Source: CAD feature listing. Evaluate the final solid. Frame: model axes, mm. Face numbers are marked on the shaded views. Round coordinates to 2 decimals unless told otherwise and drop trailing zeros. Order: outer loops, then holes, each group sorted by start corner. A loop starts at its lowest first (then second) coordinate and runs counter-clockwise, first axis right, second up. Notation, with made-up numbers: M 61.5,-10 L 91.5,-10 A32 cw 91.5,29 Z; hole C 87.25,51 d5. An arc over 180 degrees is marked long. Answer in a Markdown table with one row per item. Add a question column.
```python
from build123d import *

# Parameters (mm, degrees)
F1_DEPTH = 25.4
F2_T     = -2.54
F4_D     = 12.7


with BuildPart() as f1:
    # F0 (on Top) → F1 (new body)
    with BuildSketch(Plane.XY):
        with BuildLine():
            ThreePointArc((-34.137599, 0), (2.286002, -13.83152), (38.709603, 0))
            ThreePointArc((38.709603, 0), (2.286002, 13.957497), (-34.137599, 0))
        make_face()
    extrude(amount=F1_DEPTH)

    # F2
    f2_openings = [f1.faces().sort_by_distance(p)[0] for p in [
        (2.286002, 0.052928, 0),
    ]]
    offset(amount=F2_T, openings=f2_openings)

    # F4 (through all)
    with Locations(Plane(origin=(0, 0, 0), x_dir=(1, 0, 0), z_dir=(0, 0, -1))):
        with Locations((0, 0)):
            Hole(F4_D / 2)


solid = f1.part
```
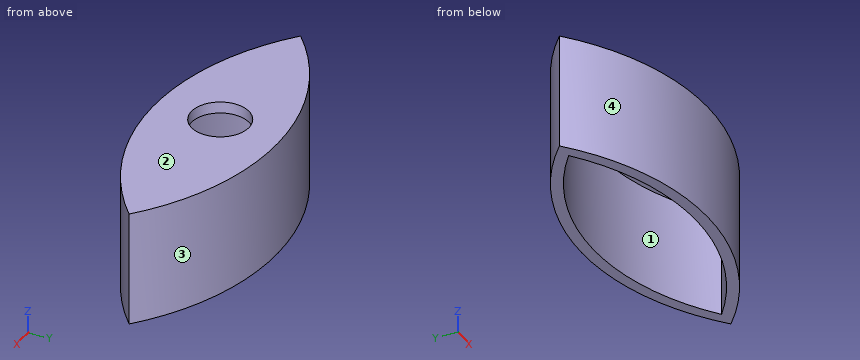
(1) Cut plane A-A (y = 3). Return loops of the section in (x, z), and give its area (3 significant figures).
(2) Cut plane D-D (x = 26). Return loops of the section in (y, z), and give its area (3 significant figures).
(3) Pin query (flat end, axial travel): pin 1 (10 mm diameter, centred on x = -7.5, y = -4.5, fed in from -Z); pin 2 (4 mm diameter, centred on x = 12, z = 13, fed in from -Y); pin 3 (7.5 mm diameter, centred on x = 0, y = 0, fed in from -Z); pin 4 (1 mm diameter, centred on y = 6, z = 16, fed in from -X). Return the tip coordinate at first contact, or that it passes through.
(4) Cut plane C-C (z = 9.25). Return loops of the section in (x, y).
(5) Cut plane B-B (x = 0). Return loops of the section in (y, z).
(6) Line query: line 1 (Z direction, x = -7, y = -2); line 2 (Y direction, x = -20, z = 14.25); line 3 (X direction, y = -5.5, z = 10.5). Output: solid intervals per line, ascending. Write a range as from..to.
(7) Draft query along Y for the marked faces 1, 2, 3 and 4. Return one class per face: +Y half, -Y half, draft (parallel to the pull), parting line (faces both ways), or undercut.
Answer list:
| question | item | result |
|---|---|---|
| 1 | outline | M -30.49,0 L -26.07,0 L -26.07,22.86 L -5.6,22.86 L -5.6,25.4 L -30.49,25.4 Z; M 5.6,22.86 L 30.64,22.86 L 30.64,0 L 35.06,0 L 35.06,25.4 L 5.6,25.4 Z |
| 1 | area | 340 mm² |
| 2 | outline | M -8.44,0 L -5.61,0 L -5.61,22.86 L 5.69,22.86 L 5.69,0 L 8.53,0 L 8.53,25.4 L -8.44,25.4 Z |
| 2 | area | 173 mm² |
| 3 | pin 1 | z = 22.86 |
| 3 | pin 2 | y = -13.29 |
| 3 | pin 3 | through |
| 3 | pin 4 | x = -26.88 |
| 4 | outline | M -34.14,0 A54.87 ccw 38.71,0 A54.5 ccw Z; hole M -30.2,0.01 A52.33 ccw 34.77,0.01 A51.96 ccw Z |
| 5 | outline | M -13.78,0 L -11.24,0 L -11.24,22.86 L -6.35,22.86 L -6.35,25.4 L -13.78,25.4 Z; M 6.35,22.86 L 11.37,22.86 L 11.37,0 L 13.91,0 L 13.91,25.4 L 6.35,25.4 Z |
| 6 | line 1 | 22.86..25.4 |
| 6 | line 2 | -9.1..-6.31, 6.4..9.19 |
| 6 | line 3 | -26.78..-21.64, 26.22..31.35 |
| 7 | face 1 | undercut |
| 7 | face 2 | draft |
| 7 | face 3 | +Y half |
| 7 | face 4 | -Y half |
